```python
from build123d import *

# Parameters (mm, degrees)
F0_R      = 50.8
F1_DEPTH  = 152.4
F2_R      = 48.661365
F3_DEPTH  = 139.7
F3_FACE_R = 48.661365
F4_DEPTH  = 139.7


with BuildPart() as f1:
    # F0 (on Front) → F1 (new body)
    with BuildSketch(Plane.XZ):
        Circle(F0_R)
    extrude(amount=F1_DEPTH)

    # F2 (on face) → F3 (cut)
    with BuildSketch(Plane.XZ.offset(152.4)):
        Circle(F2_R)
    extrude(amount=-F3_DEPTH, mode=Mode.SUBTRACT)

    # F2 (on face) + F3_face (on face) → F4 (cut)
    with BuildSketch(Plane.XZ.offset(152.4)):
        Circle(F2_R)
    with BuildSketch(Plane.XZ.offset(12.7)):
        Circle(F3_FACE_R)
    extrude(amount=-F4_DEPTH, mode=Mode.SUBTRACT)


solid = f1.part
```
Can you work these out from the model? Positions are in its coordinate system, mm. Give positions to 0.01 mm unless a question says otherwise; leave off trailing zeros. Write each loop counter-clockwise with the first axis right and the second up, starting at its lowest first coordinate (ties: lowest second). Pieces come first, ordered by that corner, then holes. Notation, with made-up numbers: (84, -29.75) - (117, -29.75) arc R32 cw to (117, 0.25) - close; hole circle Ø7 at (-2.75, 42). An arc over 180 degrees is marked (long way). Write item = value, one per line. Start each with the question number.
1. Imagine slicing it at A-A (z = 0). Please give me the cut outline in (x, y).
2. Imagine slicing it at C-C (y = -75). Please give me the cut outline in (x, z), and give its area (3 significant figures).
3. For pin 1 (4 mm diameter, centred on x = -14, y = -96, fed in from +Z); pin 2 (10 mm diameter, centred on y = -72, z = 6, fed in from +X); pin 3 (10 mm diameter, centred on x = -39, z = -3.5, fed in from +Y); pin 4 (1 mm diameter, centred on x = 29.5, y = -116.5, fed in from -Z), each with a flat end and sliding along its axis, tell me the tip position at first contact or that it passes through.
4. Imagine slicing it at B-B (x = 0). Please give me the cut outline in (y, z).
5. Thinking about a two-plate mould opening in Z: for faces 1 (the face through (-38.616, -77.267, -29.61)), 2 (the face through (-11.012, -75.133, -49.592)), 3 (the face through (0, -152.4, -49)), which applies, released by +Z, released by -Z, zero draft, split by the parting line, or undercut?
6. Please list where these lines run through material, in increasing order: line 1 (Z direction, x = 0, y = -60); line 2 (Z direction, x = -13, y = -103.5); line 3 (X direction, y = -8, z = 34).
Worked answers:
q1.outline = (-50.8, -152.4) - (-48.66, -152.4) - (-48.66, 0) - (-50.8, 0) - close; (48.66, -152.4) - (50.8, -152.4) - (50.8, 0) - (48.66, 0) - close
q2.outline = circle Ø101.6 at (0, 0); hole circle Ø97.32 at (0, 0)
q2.area = 668 mm2
q3.pin_1 = 49.36
q3.pin_2 = 50.79
q3.pin_3 = through
q3.pin_4 = -41.71
q4.outline = (-152.4, -50.8) - (0, -50.8) - (0, -48.66) - (-152.4, -48.66) - close; (-152.4, 48.66) - (0, 48.66) - (0, 50.8) - (-152.4, 50.8) - close
q5.face_1 = undercut
q5.face_2 = split by the parting line
q5.face_3 = zero draft
q6.line_1 = -50.8 to -48.66, 48.66 to 50.8
q6.line_2 = -49.11 to -46.89, 46.89 to 49.11
q6.line_3 = -37.74 to -34.81, 34.81 to 37.74
